The model under review builds one solid part; all positions refer to its coordinate system, in mm. A direction names the side the tool comes from. Give positions to 0.01 mm unless a question says otherwise; leave off trailing zeros. Order: outer loops, then holes, each group sorted by start corner. A loop starts at its lowest first (then second) coordinate and runs counter-clockwise, first axis right, second up.
```python
from build123d import *

# Parameters (mm, degrees)
BOSS_EXTRUDE1_DEPTH = 25
BOSS_EXTRUDE2_DEPTH = 15
SKETCH3_W           = 15
SKETCH3_H           = 10
CUT_EXTRUDE1_DEPTH  = 14


with BuildPart() as part:
    # Sketch1 → Boss-Extrude1 (new body)
    with BuildSketch(Plane.XY):
        Polygon((-30, 15), (-15, 15), (-15, 25), (0, 25), (0, 0), (-30, 0), align=None)
    extrude(amount=BOSS_EXTRUDE1_DEPTH)

    # Sketch2 → Boss-Extrude2 (add)
    with BuildSketch(Plane.ZY.offset(15)):
        Polygon((0, 25), (25, 15), (0, 15), align=None)
    extrude(amount=BOSS_EXTRUDE2_DEPTH)

    # Sketch3 → Cut-Extrude1 (cut)
    with BuildSketch(Plane(origin=(0, 0, 0), x_dir=(-1, 0, 0), z_dir=(0, 0, -1))):
        with Locations((22.5, 5)):
            Rectangle(SKETCH3_W, SKETCH3_H)
    extrude(amount=-CUT_EXTRUDE1_DEPTH, mode=Mode.SUBTRACT)


solid = part.part
```
1. For faces 1 (the flat face through (-15, 22, 18)), 2 (the flat face through (-22, 10, 7)), 3 (the flat face through (-30, 13, 13)), list the 3-axis set-ups (+Z, -Z, +X, -X, +Y, -Y) from which the entire face can be reached by the end or side of a thin tool; tool diameter is ignored.
2. To check wall thickness, follow line 1 (Z direction, x = -15.5, y = 4.25); line 2 (X direction, y = 9.5, z = 2.75); line 3 (Y direction, x = -25.25, z = 19). State the ranges of each line that lie inside material, in increasing order.
3. Take a section at C-C (x = -19.25). Write out the cut boundary in (y, z).
4. Take a section at B-B (y = 4.5). Write out the cut boundary in (x, z), and give its area (3 significant figures).
5. Insertion check: pin 1 (3 mm diameter, centred on y = 6, z = 18.5, fed in from +X); pin 2 (7 mm diameter, centred on x = -25.5, z = 8.5, fed in from -Y); pin 3 (6 mm diameter, centred on x = -26, z = 21, fed in from +Y); pin 4 (5 mm diameter, centred on x = -20.5, y = 7, fed in from -Z). Each pin has a flat end and moves straight along its axis. Give the tip position at first contact, or say it passes through.
6. Take a section at A-A (z = 7.5). Write out the cut boundary in (x, y), and give its area (3 significant figures).
7. Take a section at D-D (z = 3.75). Write out the cut boundary in (x, y).
Answer:
1. face 1: +Z, -X, +Y
1. face 2: -Z, -X, -Y
1. face 3: +Z, -Z, -X, +Y, -Y
2. line 1: z = 14 to 25
2. line 2: x = -15 to 0
2. line 3: y = 0 to 17.4
3. outline: (0, 14) - (10, 14) - (10, 0) - (25, 0) - (15, 25) - (0, 25) - close
4. outline: (-30, 14) - (-15, 14) - (-15, 0) - (0, 0) - (0, 25) - (-30, 25) - close
4. area: 540 mm2
5. pin 1: stops at x = 0
5. pin 2: stops at y = 10
5. pin 3: stops at y = 17.8
5. pin 4: stops at z = 14
6. outline: (-30, 10) - (-15, 10) - (-15, 0) - (0, 0) - (0, 25) - (-15, 25) - (-15, 22) - (-30, 22) - close
6. area: 555 mm2
7. outline: (-30, 10) - (-15, 10) - (-15, 0) - (0, 0) - (0, 25) - (-15, 25) - (-15, 23.5) - (-30, 23.5) - close
